from build123d import *

# Parameters (mm, degrees)
F0_W     = 25.4
F0_H     = 25.400001
F1_DEPTH = 25.4
F2_R     = 5.08
F3_R     = 5.08
F4_R     = 5.08
F5_R     = 5.08
F6_R     = 5.08


with BuildPart() as f1:
    # F0 (on Top) → F1 (new body)
    with BuildSketch(Plane.XY):
        with Locations((-4.615962, 5.455227)):
            Rectangle(F0_W, F0_H)
    extrude(amount=F1_DEPTH)

    # F2
    f2_edges = [f1.edges().sort_by_distance(p)[0] for p in [
        (-17.315962, 5.455228, 25.4),
    ]]
    fillet(f2_edges, radius=F2_R)

    # F3
    f3_edges = [f1.edges().sort_by_distance(p)[0] for p in [
        (-2.075962, 18.155228, 25.4),
    ]]
    fillet(f3_edges, radius=F3_R)

    # F4
    f4_edges = [f1.edges().sort_by_distance(p)[0] for p in [
        (8.084038, 2.915228, 25.4),
    ]]
    fillet(f4_edges, radius=F4_R)

    # F5
    f5_edges = [f1.edges().sort_by_distance(p)[0] for p in [
        (-4.615962, -7.244773, 25.4),
    ]]
    fillet(f5_edges, radius=F5_R)

    # F6
    f6_edges = [f1.edges().sort_by_distance(p)[0] for p in [
        (-4.615962, -7.244773, 0),
    ]]
    fillet(f6_edges, radius=F6_R)


solid = f1.part
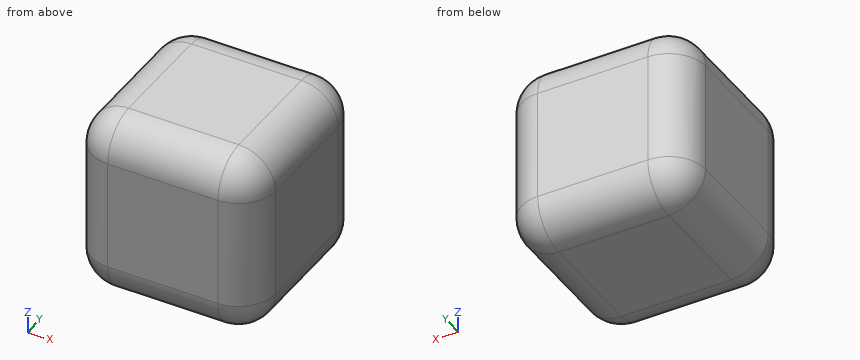
For this review, take the finished solid that the model builds, in its own axes (mm). Give positions to 0.01 mm unless a question says otherwise; leave off trailing zeros. Loops run counter-clockwise (first coordinate to the right, second up) from the corner with the lowest first, then second, coordinate; pieces in that order, holes last. Notation, with made-up numbers: M -38,25 L 21,25 A24 ccw 21,49 Z; hole C 51,3 d11. An arc over 180 degrees is marked long. Answer as a JSON object with one key per item and string values. Group by question number.
Q1. Add section A-A on x = -8.5. Give the boundary of the cut face in (y, z).
Q2. For probe 1 along Z at (x, y) = (-12.5, 4.5); probe 2 along Y at (x, z) = (-12.5, 17.25); probe 3 along X at (y, z) = (7.75, 5), list the stretches that pass through material, from the lowest coordinate up. Write a range as [from, to].
Q3. Add section B-B on y = 3.5. Give the boundary of the cut face in (x, z), and give its area (3 significant figures).
Checked values:
{
 "1": {"outline": "M -7.24,5.08 A5.08 ccw -2.16,0 L 13.08,0 A5.08 ccw 18.16,5.08 L 18.16,20.32 A5.08 ccw 13.08,25.4 L -2.16,25.4 A5.08 ccw -7.24,20.32 Z"},
 "2": {"probe 1": "[0.01, 25.39]", "probe 2": "[-7.24, 18.15]", "probe 3": "[-17.32, 8.08]"},
 "3": {"outline": "M -17.32,5.08 A5.08 ccw -12.24,0 L 3,0 A5.08 ccw 8.08,5.08 L 8.08,20.32 A5.08 ccw 3,25.4 L -12.24,25.4 A5.08 ccw -17.32,20.32 Z", "area": "623 mm²"}
}
